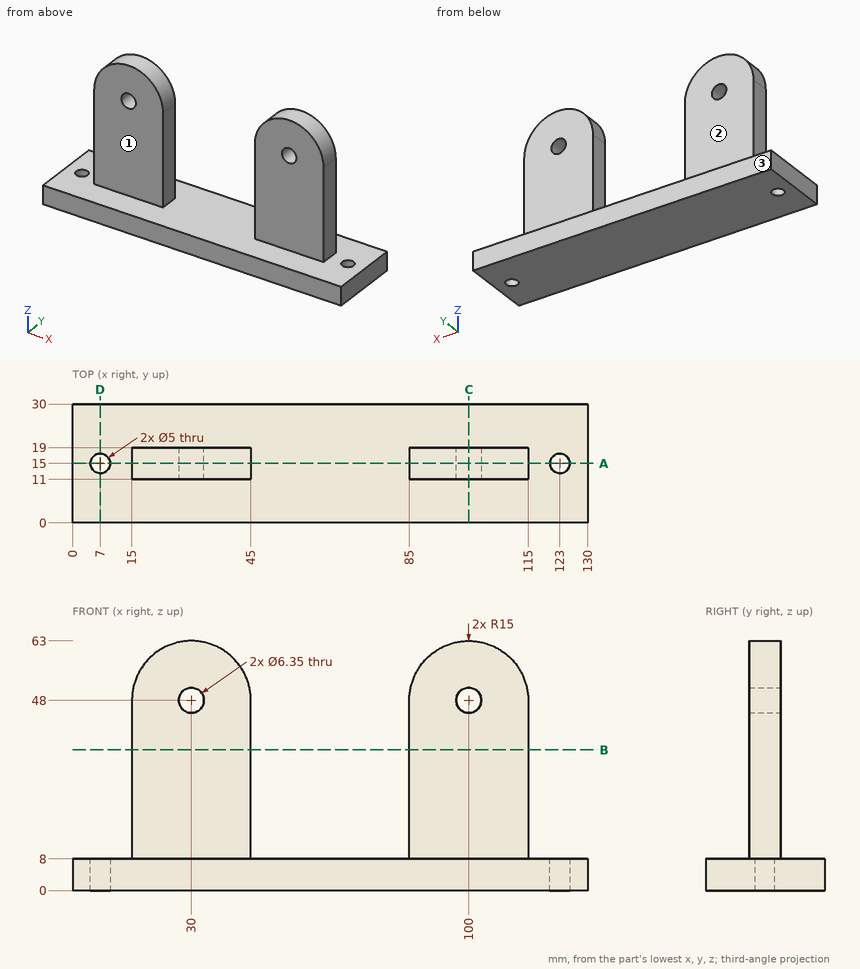
Can you work these out from the drawing? Everything is in mm from the part's minimum corner. A direction names the side the tool comes from. Coordinates: 2 decimals unless noted, no trailing zeros. Order: outer loops, then holes, each group sorted by start corner. A loop starts at its lowest first (then second) coordinate and runs counter-clockwise, first axis right, second up. Notation, with made-up numbers: (72.5, 74) -> (100.5, 74) arc R14 ccw to (100.5, 87) -> close; hole circle Ø6 at (62.5, 79). An arc over 180 degrees is marked (long way). Use one line per item in the form item = value.
Q1. I need wall thicknesses on L1, parallel to X at y = 17, z = 48 (3 decimals); L2, parallel to X at y = 15, z = 5; L3, parallel to X at y = 18.75, z = 13.5. Which ranges of each line are inside material? Lowest first, please.
From the geometry:
L1 = 15 to 26.825, 33.175 to 45, 85 to 96.825, 103.175 to 115
L2 = 0 to 4.5, 9.5 to 120.5, 125.5 to 130
L3 = 15 to 45, 85 to 115
Q2. Imagine slicing it at A-A, the plane y = 15. List the corners of the cut face in (x, z) for me (3 decimals), then the cut area to 3 significant figures.
From the geometry:
outline = (0, 0) -> (4.5, 0) -> (4.5, 8) -> (0, 8) -> close; (9.5, 0) -> (120.5, 0) -> (120.5, 8) -> (115, 8) -> (115, 48) arc R15 ccw to (85, 48) -> (85, 8) -> (45, 8) -> (45, 48) arc R15 ccw to (15, 48) -> (15, 8) -> (9.5, 8) -> close; (125.5, 0) -> (130, 0) -> (130, 8) -> (125.5, 8) -> close; hole circle Ø6.35 at (30, 48); hole circle Ø6.35 at (100, 48)
area = 4,000 mm²
Q3. Imagine slicing it at B-B, the plane z = 35.5. List the corners of the cut face in (x, y) for me, then the cut area to 3 significant figures.
From the geometry:
outline = (15, 11) -> (45, 11) -> (45, 19) -> (15, 19) -> close; (85, 11) -> (115, 11) -> (115, 19) -> (85, 19) -> close
area = 480 mm²
Q4. Imagine slicing it at C-C, the plane x = 100. List the corners of the cut face in (y, z) for me (3 decimals), then the cut area to 3 significant figures.
From the geometry:
outline = (0, 0) -> (30, 0) -> (30, 8) -> (19, 8) -> (19, 44.825) -> (11, 44.825) -> (11, 8) -> (0, 8) -> close; (11, 51.175) -> (19, 51.175) -> (19, 63) -> (11, 63) -> close
area = 629 mm²
Q5. Imagine slicing it at D-D, the plane x = 7. List the corners of the cut face in (y, z) for me, then the cut area to 3 significant figures.
From the geometry:
outline = (0, 0) -> (12.5, 0) -> (12.5, 8) -> (0, 8) -> close; (17.5, 0) -> (30, 0) -> (30, 8) -> (17.5, 8) -> close
area = 200 mm²
Q6. Will these pins go through, and if not, where does the flat tip stop? P1, Ø4, axis at x = 56, y = 12, coming from the +Z side; P2, Ø4, axis at y = 20.5, z = 44.5, coming from the +X side; P3, Ø6, axis at x = 104, z = 33.5, coming from the -Y side; P4, Ø1, axis at x = 114.5, y = 15.5, coming from the -Z side.
From the geometry:
P1 = 8
P2 = 115
P3 = 11
P4 = 0
Q7. Which directions (+Z, -Z, +X, -X, +Y, -Y) give clear straight access to the entire face, cutting with the end or side of a thin tool? Please do the marked faces 1, 2 and 3.
From the geometry:
face_1 = +Z, +X, -X, -Y
face_2 = +Z, +X, -X, +Y
face_3 = +Z, -Z, +X, -X, +Y
